Geometry: final body of the model. Coordinates: model frame, mm. A direction names the side the tool comes from. Give positions to 0.01 mm unless a question says otherwise; leave off trailing zeros. Order: outer loops, then holes, each group sorted by start corner. A loop starts at its lowest first (then second) coordinate and runs counter-clockwise, first axis right, second up. Notation, with made-up numbers: (-8.5, -28.5) - (46.5, -28.5) arc R12 ccw to (46.5, -22.5) - close; hole circle Ø7 at (49, 65). An arc over 180 degrees is marked (long way). One line per item, written item: value.
```python
from build123d import *

# Parameters (mm, degrees)
F1_DEPTH = 25.4
F2_R     = 3.175
F4_DEPTH = 32.259
F5_R     = 6.35
F6_R     = 3.175


with BuildPart() as f1:
    # F0 (on Top) → F1 (new body)
    with BuildSketch(Plane.XY):
        Polygon((-30.5435, 29.083), (0, 29.083), (30.5435, 29.083), (30.5435, 0), (59.1185, 0), (59.1185, 3.175), (33.7185, 3.175), (33.7185, 32.258), (0, 32.258), (-33.7185, 32.258), (-33.7185, 3.175), (-59.1185, 3.175), (-59.1185, 0), (-30.5435, 0), align=None)
    extrude(amount=F1_DEPTH)

    # F2
    f2_edges = [f1.edges().sort_by_distance(p)[0] for p in [
        (-30.5435, 0, 12.7),
        (30.5435, 0, 12.7),
    ]]
    fillet(f2_edges, radius=F2_R)

    # F3 (on Front) → F4 (cut, through all)
    with BuildSketch(Plane.XZ):
        with BuildLine():
            ThreePointArc((-48.8315, 7.8105), (-46.4185, 5.3975), (-44.0055, 7.8105))
            Line((-44.0055, 7.8105), (-44.0055, 17.4625))
            ThreePointArc((-44.0055, 17.4625), (-46.4185, 19.8755), (-48.8315, 17.4625))
            Line((-48.8315, 17.4625), (-48.8315, 7.8105))
        make_face()
        with BuildLine():
            Line((44.0055, 17.4625), (44.0055, 7.8105))
            ThreePointArc((44.0055, 7.8105), (46.4185, 5.3975), (48.8315, 7.8105))
            Line((48.8315, 7.8105), (48.8315, 17.4625))
            ThreePointArc((48.8315, 17.4625), (46.4185, 19.8755), (44.0055, 17.4625))
        make_face()
    extrude(amount=-F4_DEPTH, mode=Mode.SUBTRACT)

    # F5
    f5_edges = [f1.edges().sort_by_distance(p)[0] for p in [
        (-59.1185, 1.5875, 0),
        (-59.1185, 1.5875, 25.4),
        (59.1185, 1.5875, 25.4),
        (59.1185, 1.5875, 0),
    ]]
    fillet(f5_edges, radius=F5_R)

    # F6
    f6_edges = [f1.edges().sort_by_distance(p)[0] for p in [
        (-33.7185, 3.175, 12.7),
        (-33.7185, 32.258, 12.7),
        (33.7185, 32.258, 12.7),
        (33.7185, 3.175, 12.7),
    ]]
    fillet(f6_edges, radius=F6_R)


solid = f1.part
```
1) Mould query, pull axis X, two halves, no side actions, for faces 6 (the face through (0, 29.083, 13)), 7 (the face through (-46.5, 1.6, 5.4)), 8 (the face through (57.2, 1.6, 23.6)), 9 (the face through (-32.764, 31.353, 12.878)). Classes: released by +X, released by -X, zero draft, split by the parting line, or undercut.
Answers below:
face 6: undercut
face 7: undercut
face 8: released by +X
face 9: released by -X
2) Section A-A, the plane z = 14.5. Count the separate pieces of the cut face and the enclosed holes in it, then the cut area to 3 significant figures.
Answers below:
separate pieces: 3
enclosed holes: 0
area: 525 mm^2
3) Section B-B, the plane y = 10.5. Return loops of the section in (x, z).
Answers below:
outline: (-33.72, 0) - (-30.54, 0) - (-30.54, 25.4) - (-33.72, 25.4) - close; (30.54, 0) - (33.72, 0) - (33.72, 25.4) - (30.54, 25.4) - close
4) Section D-D, the plane y = 4.5. Return loops of the section in (x, z).
Answers below:
outline: (-34.31, 0) - (-30.54, 0) - (-30.54, 25.4) - (-34.31, 25.4) - close; (30.54, 0) - (34.31, 0) - (34.31, 25.4) - (30.54, 25.4) - close
5) Material intervals for line 1 along X through (y, z) = (26.5, 16); line 2 along Y through (x, z) = (-9.5, 3.5); line 3 along Y through (x, z) = (-52.5, 14.25) (3 decimals), sorted ascending.
Answers below:
line 1: -33.72 to -30.54, 30.54 to 33.72
line 2: 29.08 to 32.26
line 3: 0 to 3.175
6) Section C-C, the plane x = 22. Return loops of the section in (y, z), then the cut area to 3 significant figures.
Answers below:
outline: (29.08, 0) - (32.26, 0) - (32.26, 25.4) - (29.08, 25.4) - close
area: 80.6 mm^2
7) Set-up query: faces 1 (the face through (33.718, 18, 13)), 2 (the face through (-59.118, 2, 13)), 3 (the face through (-31.498, 0.905, 12.878)), 4 (the face through (-57.2, 1.6, 23.6)), 5 (the face through (46.365, 1.565, 5.398)). Return all of +Z, -Z, +X, -X, +Y, -Y with unobstructed straight access to the full face (end or side cutting, diameter ignored); none if empty.
Answers below:
face 1: +Z, -Z, +X, +Y
face 2: +Z, -Z, -X, +Y, -Y
face 3: +Z, -Z, -Y
face 4: +Z, -X, +Y, -Y
face 5: +Y, -Y
8) First-contact query: pin 1 (4 mm diameter, centred on y = 10.5, z = 3.5, fed in from -X); pin 2 (2 mm diameter, centred on x = 29, z = 20.5, fed in from -Y); pin 3 (12.5 mm diameter, centred on y = 17, z = 12.5, fed in from +X). Flat tips, straight axial feed; report the tip coordinate or a pass-through.
Answers below:
pin 1: x = -33.72
pin 2: y = 29.08
pin 3: x = 33.72
